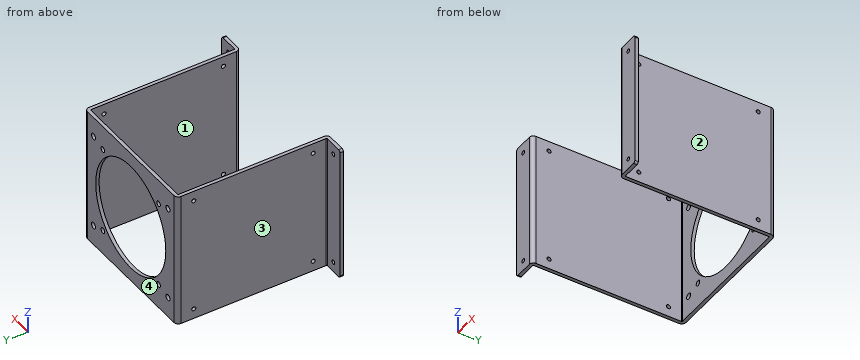
```python
from build123d import *

# Parameters (mm, degrees)
BASE_FLANGE1_START = -100
BASE_FLANGE1_DEPTH = 200
CUT_EXTRUDE1_REACH = 282.802
SKETCH6_R          = 3
CUT_EXTRUDE2_REACH = 282.802
SKETCH7_R          = 80
SKETCH7_R_2        = 4
CUT_EXTRUDE3_REACH = 345.839
SKETCH8_R          = 3
FILLET1_R          = 3
CUT_EXTRUDE4_REACH = 282.802
SKETCH9_R          = 4.5


# Read off the part's stored shape, not the designer's step: Base-Flange1
with BuildPart() as part:
    # Base-Flange1 outline → Base-Flange1 (new body)
    with BuildSketch(Plane.XY.offset(BASE_FLANGE1_START)):
        with BuildLine():
            Line((-106, 5), (-135, 5))
            Line((-135, 5), (-135, 0))
            Line((-135, 0), (-106, 0))
            ThreePointArc((-106, 0), (-101.757359313, 1.757359313), (-100, 6))
            Line((-100, 6), (-100, 219))
            ThreePointArc((-100, 219), (-99.707106781, 219.707106781), (-99, 220))
            Line((-99, 220), (99, 220))
            ThreePointArc((99, 220), (99.707106781, 219.707106781), (100, 219))
            Line((100, 219), (100, 6))
            ThreePointArc((100, 6), (101.757359313, 1.757359313), (106, 0))
            Line((106, 0), (135, 0))
            Line((135, 0), (135, 5))
            Line((135, 5), (106, 5))
            ThreePointArc((106, 5), (105.292893219, 5.292893219), (105, 6))
            Line((105, 6), (105, 219))
            ThreePointArc((105, 219), (103.242640687, 223.242640687), (99, 225))
            Line((99, 225), (-99, 225))
            ThreePointArc((-99, 225), (-103.242640687, 223.242640687), (-105, 219))
            Line((-105, 219), (-105, 6))
            ThreePointArc((-105, 6), (-105.292893219, 5.292893219), (-106, 5))
        make_face()
    extrude(amount=BASE_FLANGE1_DEPTH)

    # Sketch6 → Cut-Extrude1 (cut, up to next)
    with BuildSketch(Plane.XZ, mode=Mode.PRIVATE) as cut_extrude1_sk1:
        with Locations((-120, 85)):
            Circle(SKETCH6_R)
    cut_extrude1_tool1 = extrude(cut_extrude1_sk1.sketch, amount=-CUT_EXTRUDE1_REACH, mode=Mode.PRIVATE) & part.part
    # Sketch6 → Cut-Extrude1 (cut, up to next)
    with BuildSketch(Plane.XZ, mode=Mode.PRIVATE) as cut_extrude1_sk2:
        with Locations((120, 85)):
            Circle(SKETCH6_R)
    cut_extrude1_tool2 = extrude(cut_extrude1_sk2.sketch, amount=-CUT_EXTRUDE1_REACH, mode=Mode.PRIVATE) & part.part
    # Sketch6 → Cut-Extrude1 (cut, up to next)
    with BuildSketch(Plane.XZ, mode=Mode.PRIVATE) as cut_extrude1_sk3:
        with Locations((120, -85)):
            Circle(SKETCH6_R)
    cut_extrude1_tool3 = extrude(cut_extrude1_sk3.sketch, amount=-CUT_EXTRUDE1_REACH, mode=Mode.PRIVATE) & part.part
    # Sketch6 → Cut-Extrude1 (cut, up to next)
    with BuildSketch(Plane.XZ, mode=Mode.PRIVATE) as cut_extrude1_sk4:
        with Locations((-120, -85)):
            Circle(SKETCH6_R)
    cut_extrude1_tool4 = extrude(cut_extrude1_sk4.sketch, amount=-CUT_EXTRUDE1_REACH, mode=Mode.PRIVATE) & part.part
    add(cut_extrude1_tool1.solids().sort_by_distance((-120, 0, 85))[0], mode=Mode.SUBTRACT)
    add(cut_extrude1_tool2.solids().sort_by_distance((120, 0, 85))[0], mode=Mode.SUBTRACT)
    add(cut_extrude1_tool3.solids().sort_by_distance((120, 0, -85))[0], mode=Mode.SUBTRACT)
    add(cut_extrude1_tool4.solids().sort_by_distance((-120, 0, -85))[0], mode=Mode.SUBTRACT)

    # Sketch7 → Cut-Extrude2 (cut, up to next)
    with BuildSketch(Plane(origin=(0, 225, 0), x_dir=(1, 0, 0), z_dir=(0, 1, 0)), mode=Mode.PRIVATE) as cut_extrude2_sk1:
        with Locations(Location((0, 0, 0), (0, 0, 180))):
            Circle(SKETCH7_R)
    cut_extrude2_tool1 = extrude(cut_extrude2_sk1.sketch, amount=-CUT_EXTRUDE2_REACH, mode=Mode.PRIVATE) & part.part
    # Sketch7 → Cut-Extrude2 (cut, up to next)
    with BuildSketch(Plane(origin=(0, 225, 0), x_dir=(1, 0, 0), z_dir=(0, 1, 0)), mode=Mode.PRIVATE) as cut_extrude2_sk2:
        with Locations(Location((-63.639610307, 63.639610307, 0), (0, 0, 180))):
            Circle(SKETCH7_R_2)
    cut_extrude2_tool2 = extrude(cut_extrude2_sk2.sketch, amount=-CUT_EXTRUDE2_REACH, mode=Mode.PRIVATE) & part.part
    # Sketch7 → Cut-Extrude2 (cut, up to next)
    with BuildSketch(Plane(origin=(0, 225, 0), x_dir=(1, 0, 0), z_dir=(0, 1, 0)), mode=Mode.PRIVATE) as cut_extrude2_sk3:
        with Locations((63.639610307, 63.639610307)):
            Circle(SKETCH7_R_2)
    cut_extrude2_tool3 = extrude(cut_extrude2_sk3.sketch, amount=-CUT_EXTRUDE2_REACH, mode=Mode.PRIVATE) & part.part
    # Sketch7 → Cut-Extrude2 (cut, up to next)
    with BuildSketch(Plane(origin=(0, 225, 0), x_dir=(1, 0, 0), z_dir=(0, 1, 0)), mode=Mode.PRIVATE) as cut_extrude2_sk4:
        with Locations(Location((63.639610307, -63.639610307, 0), (0, 0, 180))):
            Circle(SKETCH7_R_2)
    cut_extrude2_tool4 = extrude(cut_extrude2_sk4.sketch, amount=-CUT_EXTRUDE2_REACH, mode=Mode.PRIVATE) & part.part
    # Sketch7 → Cut-Extrude2 (cut, up to next)
    with BuildSketch(Plane(origin=(0, 225, 0), x_dir=(1, 0, 0), z_dir=(0, 1, 0)), mode=Mode.PRIVATE) as cut_extrude2_sk5:
        with Locations((-63.639610307, -63.639610307)):
            Circle(SKETCH7_R_2)
    cut_extrude2_tool5 = extrude(cut_extrude2_sk5.sketch, amount=-CUT_EXTRUDE2_REACH, mode=Mode.PRIVATE) & part.part
    add(cut_extrude2_tool1.solids().sort_by_distance((0, 225, 0))[0], mode=Mode.SUBTRACT)
    add(cut_extrude2_tool2.solids().sort_by_distance((-63.63961, 225, -63.63961))[0], mode=Mode.SUBTRACT)
    add(cut_extrude2_tool3.solids().sort_by_distance((63.63961, 225, -63.63961))[0], mode=Mode.SUBTRACT)
    add(cut_extrude2_tool4.solids().sort_by_distance((63.63961, 225, 63.63961))[0], mode=Mode.SUBTRACT)
    add(cut_extrude2_tool5.solids().sort_by_distance((-63.63961, 225, 63.63961))[0], mode=Mode.SUBTRACT)

    # Cut-Extrude3: up to this face of the body (flat: up to its plane)
    cut_extrude3_end = Plane(part.part.faces().sort_by_distance((-105, 112.5, 0))[0])
    # Sketch8 → Cut-Extrude3 (cut, up to the picked face)
    with BuildSketch(Plane(origin=(105, 0, 0), x_dir=(0, 0, -1), z_dir=(1, 0, 0)), mode=Mode.PRIVATE) as cut_extrude3_sk1:
        with Locations(Location((85, 200, 0), (0, 0, 90))):
            Circle(SKETCH8_R)
    cut_extrude3_tool1 = split(extrude(cut_extrude3_sk1.sketch, amount=-CUT_EXTRUDE3_REACH, mode=Mode.PRIVATE), bisect_by=cut_extrude3_end, keep=Keep.BOTH, mode=Mode.PRIVATE)
    # Sketch8 → Cut-Extrude3 (cut, up to the picked face)
    with BuildSketch(Plane(origin=(105, 0, 0), x_dir=(0, 0, -1), z_dir=(1, 0, 0)), mode=Mode.PRIVATE) as cut_extrude3_sk2:
        with Locations(Location((85, 25, 0), (0, 0, 90))):
            Circle(SKETCH8_R)
    cut_extrude3_tool2 = split(extrude(cut_extrude3_sk2.sketch, amount=-CUT_EXTRUDE3_REACH, mode=Mode.PRIVATE), bisect_by=cut_extrude3_end, keep=Keep.BOTH, mode=Mode.PRIVATE)
    # Sketch8 → Cut-Extrude3 (cut, up to the picked face)
    with BuildSketch(Plane(origin=(105, 0, 0), x_dir=(0, 0, -1), z_dir=(1, 0, 0)), mode=Mode.PRIVATE) as cut_extrude3_sk3:
        with Locations(Location((-85, 25, 0), (0, 0, 90))):
            Circle(SKETCH8_R)
    cut_extrude3_tool3 = split(extrude(cut_extrude3_sk3.sketch, amount=-CUT_EXTRUDE3_REACH, mode=Mode.PRIVATE), bisect_by=cut_extrude3_end, keep=Keep.BOTH, mode=Mode.PRIVATE)
    # Sketch8 → Cut-Extrude3 (cut, up to the picked face)
    with BuildSketch(Plane(origin=(105, 0, 0), x_dir=(0, 0, -1), z_dir=(1, 0, 0)), mode=Mode.PRIVATE) as cut_extrude3_sk4:
        with Locations(Location((-85, 200, 0), (0, 0, 90))):
            Circle(SKETCH8_R)
    cut_extrude3_tool4 = split(extrude(cut_extrude3_sk4.sketch, amount=-CUT_EXTRUDE3_REACH, mode=Mode.PRIVATE), bisect_by=cut_extrude3_end, keep=Keep.BOTH, mode=Mode.PRIVATE)
    add(cut_extrude3_tool1.solids().sort_by(Axis((105, 200, -85), (-1, 0, 0)))[0], mode=Mode.SUBTRACT)
    add(cut_extrude3_tool2.solids().sort_by(Axis((105, 25, -85), (-1, 0, 0)))[0], mode=Mode.SUBTRACT)
    add(cut_extrude3_tool3.solids().sort_by(Axis((105, 25, 85), (-1, 0, 0)))[0], mode=Mode.SUBTRACT)
    add(cut_extrude3_tool4.solids().sort_by(Axis((105, 200, 85), (-1, 0, 0)))[0], mode=Mode.SUBTRACT)

    # Fillet1
    fillet1_edges = [part.edges().sort_by_distance(p)[0] for p in [
        (135, 2.5, -100),
        (-135, 2.5, -100),
        (135, 2.5, 100),
        (-135, 2.5, 100),
    ]]
    fillet(fillet1_edges, radius=FILLET1_R)

    # Sketch9 → Cut-Extrude4 (cut, up to next)
    with BuildSketch(Plane(origin=(0, 225, 0), x_dir=(1, 0, 0), z_dir=(0, 1, 0)), mode=Mode.PRIVATE) as cut_extrude4_sk1:
        with Locations(Location((-85, 70, 0), (0, 0, 180))):
            Circle(SKETCH9_R)
    cut_extrude4_tool1 = extrude(cut_extrude4_sk1.sketch, amount=-CUT_EXTRUDE4_REACH, mode=Mode.PRIVATE) & part.part
    # Sketch9 → Cut-Extrude4 (cut, up to next)
    with BuildSketch(Plane(origin=(0, 225, 0), x_dir=(1, 0, 0), z_dir=(0, 1, 0)), mode=Mode.PRIVATE) as cut_extrude4_sk2:
        with Locations((85, 70)):
            Circle(SKETCH9_R)
    cut_extrude4_tool2 = extrude(cut_extrude4_sk2.sketch, amount=-CUT_EXTRUDE4_REACH, mode=Mode.PRIVATE) & part.part
    # Sketch9 → Cut-Extrude4 (cut, up to next)
    with BuildSketch(Plane(origin=(0, 225, 0), x_dir=(1, 0, 0), z_dir=(0, 1, 0)), mode=Mode.PRIVATE) as cut_extrude4_sk3:
        with Locations(Location((85, -70, 0), (0, 0, 180))):
            Circle(SKETCH9_R)
    cut_extrude4_tool3 = extrude(cut_extrude4_sk3.sketch, amount=-CUT_EXTRUDE4_REACH, mode=Mode.PRIVATE) & part.part
    # Sketch9 → Cut-Extrude4 (cut, up to next)
    with BuildSketch(Plane(origin=(0, 225, 0), x_dir=(1, 0, 0), z_dir=(0, 1, 0)), mode=Mode.PRIVATE) as cut_extrude4_sk4:
        with Locations((-85, -70)):
            Circle(SKETCH9_R)
    cut_extrude4_tool4 = extrude(cut_extrude4_sk4.sketch, amount=-CUT_EXTRUDE4_REACH, mode=Mode.PRIVATE) & part.part
    add(cut_extrude4_tool1.solids().sort_by_distance((-85, 225, -70))[0], mode=Mode.SUBTRACT)
    add(cut_extrude4_tool2.solids().sort_by_distance((85, 225, -70))[0], mode=Mode.SUBTRACT)
    add(cut_extrude4_tool3.solids().sort_by_distance((85, 225, 70))[0], mode=Mode.SUBTRACT)
    add(cut_extrude4_tool4.solids().sort_by_distance((-85, 225, 70))[0], mode=Mode.SUBTRACT)


solid = part.part
```
Here's how the part is built. I have some questions about the finished solid (model axes, mm). Face numbers are marked on the shaded views. Give positions to 0.01 mm unless a question says otherwise; leave off trailing zeros. Write each loop counter-clockwise with the first axis right and the second up, starting at its lowest first coordinate (ties: lowest second). Pieces come first, ordered by that corner, then holes.
(1) Thinking about a two-plate mould opening in X: for the marked faces 1, 2, 3 and 4, which applies, pulls with the +X half, pulls with the -X half, needs draft (parallel to the pull), parting line crosses it, or undercut?
Output values:
face 1: undercut
face 2: pulls with the +X half
face 3: pulls with the -X half
face 4: needs draft
(2) Imagine slicing it at B-B, the plane z = 0. Write out the boundary of the cut face in (x, y).
Output values:
outline: (-135, 0) - (-106, 0) arc R6 ccw to (-100, 6) - (-100, 219) arc R1 cw to (-99, 220) - (-80, 220) - (-80, 225) - (-99, 225) arc R6 ccw to (-105, 219) - (-105, 6) arc R1 cw to (-106, 5) - (-135, 5) - close; (80, 220) - (99, 220) arc R1 cw to (100, 219) - (100, 6) arc R6 ccw to (106, 0) - (135, 0) - (135, 5) - (106, 5) arc R1 cw to (105, 6) - (105, 219) arc R6 ccw to (99, 225) - (80, 225) - close
(3) Imagine slicing it at D-D, the plane x = -85. Write out the boundary of the cut face in (y, z), and give its area (3 significant figures).
Output values:
outline: (220, -100) - (225, -100) - (225, -74.5) - (220, -74.5) - close; (220, -65.5) - (225, -65.5) - (225, 65.5) - (220, 65.5) - close; (220, 74.5) - (225, 74.5) - (225, 100) - (220, 100) - close
area: 910 mm2
(4) Imagine slicing it at C-C, the plane y = 78.5. Write out the boundary of the cut face in (x, z).
Output values:
outline: (-105, -100) - (-100, -100) - (-100, 100) - (-105, 100) - close; (100, -100) - (105, -100) - (105, 100) - (100, 100) - close
(5) If I drill on L1, parallel to Z at x = 101.9, y = 200; L2, parallel to X at y = 15, z = 70; L3, parallel to Z at x = 0, y = 221.1, over which ranges is the centre line in solid material (lowest first)?
Output values:
L1: z = -100 to -88, -82 to 82, 88 to 100
L2: x = -105 to -100, 100 to 105
L3: z = -100 to -80, 80 to 100
(6) Will these pins go through, and if not, where does the flat tip stop? pin 1 (1.5 mm diameter, centred on x = -96, z = -16.5, fed in from -Y); pin 2 (6 mm diameter, centred on y = 36, z = 35, fed in from -X); pin 3 (23 mm diameter, centred on x = 126, z = 13, fed in from +Y).
Output values:
pin 1: stops at y = 220
pin 2: stops at x = -105
pin 3: stops at y = 5
(7) Imagine slicing it at A-A, the plane x = 0. Write out the boundary of the cut face in (y, z), and give its area (3 significant figures).
Output values:
outline: (220, -100) - (225, -100) - (225, -80) - (220, -80) - close; (220, 80) - (225, 80) - (225, 100) - (220, 100) - close
area: 200 mm2
